Design review of the part built by this model. Coordinates are the model's own, in mm. Face numbers are marked on the shaded views. A direction names the side the tool comes from. Give positions to 0.01 mm unless a question says otherwise; leave off trailing zeros. Order: outer loops, then holes, each group sorted by start corner. A loop starts at its lowest first (then second) coordinate and runs counter-clockwise, first axis right, second up.
```python
from build123d import *

# Parameters (mm, degrees)
SKETCH3_R           = 75
BOSS_EXTRUDE1_DEPTH = 250
SKETCH4_R           = 22.984114262
CUT_EXTRUDE1_DEPTH  = 478.138344718


with BuildPart() as part:
    # Sketch3 → Boss-Extrude1 (new body)
    with BuildSketch(Plane(origin=(0, 0, 0), x_dir=(1, 0, 0), z_dir=(0, 1, 0))):
        with BuildLine():
            Line((-325, 138), (-325, 106))
            Line((-325, 106), (-145.602197786, 106))
            ThreePointArc((-145.602197786, 106), (-104.386691617, 84.306925854), (-98.9348267, 38.051282051))
            ThreePointArc((-98.9348267, 38.051282051), (0, -106), (98.9348267, 38.051282051))
            ThreePointArc((98.9348267, 38.051282051), (104.386691617, 84.306925854), (145.602197786, 106))
            Line((145.602197786, 106), (325, 106))
            Line((325, 106), (325, 138))
            Line((325, 138), (-325, 138))
        make_face()
        with Locations(Location((0, 0, 0), (0, 0, 270))):
            Circle(SKETCH3_R, mode=Mode.SUBTRACT)
    extrude(amount=BOSS_EXTRUDE1_DEPTH)

    # Sketch4 → Cut-Extrude1 (cut, through all)
    with BuildSketch(Plane(origin=(0, 0, -138), x_dir=(-1, 0, 0), z_dir=(0, 0, -1))):
        with Locations((-250, 187.5)):
            Circle(SKETCH4_R)
        with Locations((250, 187.5)):
            Circle(SKETCH4_R)
        with Locations((250, 62.5)):
            Circle(SKETCH4_R)
        with Locations((-250, 62.5)):
            Circle(SKETCH4_R)
    extrude(amount=-CUT_EXTRUDE1_DEPTH, mode=Mode.SUBTRACT)


solid = part.part
```
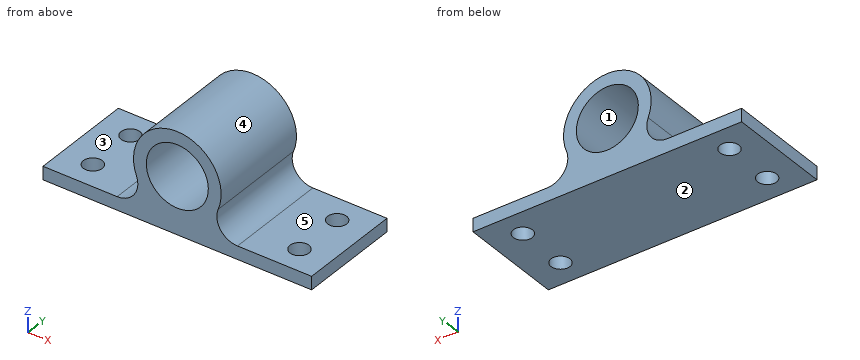
1. Draft analysis for pull direction Z (two halves, no side actions). For the marked faces 1, 2 and 3, state which applies: pulls with the +Z half, pulls with the -Z half, needs draft (parallel to the pull), parting line crosses it, or undercut.
Recorded:
face 1: undercut
face 2: pulls with the -Z half
face 3: pulls with the +Z half
2. For line 1 along Y through (x, z) = (-250, -118.5); line 2 along X through (y, z) = (125, 0); line 3 along X through (y, z) = (187, -116), list the stretches that pass through material, from the lowest coordinate up.
Recorded:
line 1: y = 0 to 39.52, 85.48 to 164.52, 210.48 to 250
line 2: x = -106 to -75, 75 to 106
line 3: x = -325 to -272.98, -227.02 to 227.02, 272.98 to 325
3. Take a section at B-B (z = 0). State the section outline as (x, y) points.
Recorded:
outline: (-106, 0) - (-75, 0) - (-75, 250) - (-106, 250) - close; (75, 0) - (106, 0) - (106, 250) - (75, 250) - close
4. For pin 1 (4 mm diameter, centred on x = 137.5, y = 46, fed in from +Z); pin 2 (4 mm diameter, centred on x = -229.5, y = 148, fed in from +Z); pin 3 (1.5 mm diameter, centred on y = 202.5, z = -10.5, fed in from -X), all flat-tipped, find the tip position at first contact; note any pin that passes through.
Recorded:
pin 1: stops at z = -104.97
pin 2: stops at z = -106
pin 3: stops at x = -105.55
5. Take a section at A-A (x = 0). State the section outline as (y, z) points, then the cut area to 3 significant figures.
Recorded:
outline: (0, -138) - (250, -138) - (250, -75) - (0, -75) - close; (0, 75) - (250, 75) - (250, 106) - (0, 106) - close
area: 23,500 mm2
6. Take a section at D-D (x = -250). State the section outline as (y, z) points.
Recorded:
outline: (0, -138) - (39.52, -138) - (39.52, -106) - (0, -106) - close; (85.48, -138) - (164.52, -138) - (164.52, -106) - (85.48, -106) - close; (210.48, -138) - (250, -138) - (250, -106) - (210.48, -106) - close
7. Take a section at C-C (y = 187.5). State the section outline as (x, z) points.
Recorded:
outline: (-325, -138) - (-272.98, -138) - (-272.98, -106) - (-325, -106) - close; (-227.02, -138) - (227.02, -138) - (227.02, -106) - (145.6, -106) arc R50 cw to (98.93, -38.05) arc R106 ccw (long way) to (-98.93, -38.05) arc R50 cw to (-145.6, -106) - (-227.02, -106) - close; (272.98, -138) - (325, -138) - (325, -106) - (272.98, -106) - close; hole circle Ø150 at (0, 0)
8. Machinability: for the marked faces 4 and 5, which of the approach directions +Z, -Z, +X, -X, +Y, -Y give a long, thin tool a straight path to every point of the face, cutting with its end or side? Answer none if there is none.
Recorded:
face 4: +Y, -Y
face 5: +Z, +X, +Y, -Y
